Read the model definition and answer for the solid it produces. Units are mm, in the model's axes. Give positions to 0.01 mm unless a question says otherwise; leave off trailing zeros. Order: outer loops, then holes, each group sorted by start corner. A loop starts at its lowest first (then second) coordinate and runs counter-clockwise, first axis right, second up. Notation, with made-up numbers: (31.5, -3) -> (84.5, -3) arc R28 cw to (84.5, 22) -> close; hole circle Ø3 at (56, 47). An arc over 180 degrees is marked (long way). Answer as CSV lines item,"result". Start each with the question number.
1) Find section A-A (y = -259.5). Determine the outline of the cut face in (x, z), and give its area (3 significant figures).
2) Straight lines are drawn through the part: L1, parallel to X at y = -383, z = -5.25; L2, parallel to Z at x = -2, y = -76; L3, parallel to Z at x = -6.25, y = -348.5. For each, find the intervals that lie inside material, in ascending order. Write a range as from..to.
3) A flat-ended cylindrical pin translates along its axis: pin 1 Ø1 at (y, z) = (-116, -5) entering from -X. Find the tip coordinate at first contact, or state that the pin passes through.
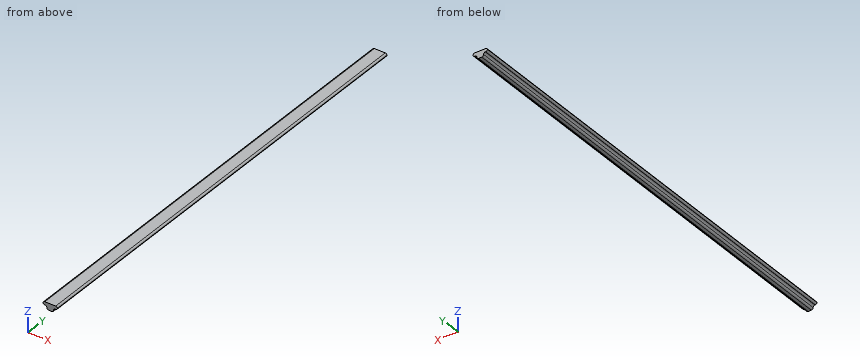
```python
from build123d import *

# Parameters (mm, degrees)
F1_DEPTH    = 500.5
F2_T1_DEPTH = 500.5
F2_T3_DEPTH = 510.5


# Not quite as in the source:
# - a fillet or chamfer that OpenCascade refuses, or shapes differently, is made with other operations: its cross-section is extruded or revolved along the edge and cut away or added


with BuildPart() as f1:
    # F0 (on Front) → F1 (new body)
    with BuildSketch(Plane.XZ):
        Polygon((8, 0), (0, 0), (-8, 0), (-8, -3.5), (-3.75, -3.5), (-3.75, -7.5), (3.75, -7.5), (3.75, -3.5), (8, -3.5), align=None)
    extrude(amount=F1_DEPTH)

    # F2: fillet of radius 2 on 8 edges, made by hand

    # F2_s2 → F2_t1 (join)
    with BuildSketch(Plane.XZ):
        with BuildLine():
            ThreePointArc((5.75, -3.5), (4.3357864376, -4.0857864376), (3.75, -5.5))
            Line((3.75, -5.5), (3.75, -3.5))
            Line((3.75, -3.5), (5.75, -3.5))
        make_face()
        with BuildLine():
            ThreePointArc((-3.75, -5.5), (-4.3357864376, -4.0857864376), (-5.75, -3.5))
            Line((-5.75, -3.5), (-3.75, -3.5))
            Line((-3.75, -3.5), (-3.75, -5.5))
        make_face()
    extrude(amount=F2_T1_DEPTH)

    # F2_s4 → F2_t3 (cut)
    with BuildSketch(Plane.XZ.offset(-5)):
        with BuildLine():
            ThreePointArc((1.75, -7.5), (3.1642135624, -6.9142135624), (3.75, -5.5))
            Line((3.75, -5.5), (3.75, -7.5))
            Line((3.75, -7.5), (1.75, -7.5))
        make_face()
        with BuildLine():
            ThreePointArc((-3.75, -5.5), (-3.1642135624, -6.9142135624), (-1.75, -7.5))
            Line((-1.75, -7.5), (-3.75, -7.5))
            Line((-3.75, -7.5), (-3.75, -5.5))
        make_face()
        with BuildLine():
            ThreePointArc((-8, -1.5), (-7.4142135624, -2.9142135624), (-6, -3.5))
            Line((-6, -3.5), (-8, -3.5))
            Line((-8, -3.5), (-8, -1.5))
        make_face()
        with BuildLine():
            ThreePointArc((-6, 0), (-7.4142135624, -0.5857864376), (-8, -2))
            Line((-8, -2), (-8, 0))
            Line((-8, 0), (-6, 0))
        make_face()
        with BuildLine():
            ThreePointArc((8, -1.5), (7.4142135624, -2.9142135624), (6, -3.5))
            Line((6, -3.5), (8, -3.5))
            Line((8, -3.5), (8, -1.5))
        make_face()
        with BuildLine():
            ThreePointArc((6, 0), (7.4142135624, -0.5857864376), (8, -2))
            Line((8, -2), (8, 0))
            Line((8, 0), (6, 0))
        make_face()
    extrude(amount=F2_T3_DEPTH, mode=Mode.SUBTRACT)


solid = f1.part
```
Findings below:
1,outline,"(-7.98, -1.75) arc R2 ccw to (-6, -3.5) -> (-5.75, -3.5) arc R2 cw to (-3.75, -5.5) arc R2 ccw to (-1.75, -7.5) -> (1.75, -7.5) arc R2 ccw to (3.75, -5.5) arc R2 cw to (5.75, -3.5) -> (6, -3.5) arc R2 ccw to (7.98, -1.75) arc R2 ccw to (6, 0) -> (-6, 0) arc R2 ccw to start"
1,area,"82.6 mm²"
2,L1,"-3.77..3.77"
2,L2,"-7.48..0"
2,L3,"-3.48..-0.02"
3,pin 1,"x = -4.02"
